from build123d import *

# Parameters (mm, degrees)
SKETCH2_W           = 203.2
SKETCH2_H           = 152.4
BOSS_EXTRUDE1_DEPTH = 152.4
SKETCH6_R           = 50.8
CUT_EXTRUDE2_DEPTH  = 228.6
SKETCH7_W           = 50.8
SKETCH7_H           = 50.8
CUT_EXTRUDE3_DEPTH  = 50.8
SKETCH5_W           = 50.8
SKETCH5_H           = 152.4
BOSS_EXTRUDE3_DEPTH = 50.8
SKETCH3_W           = 152.4
SKETCH3_H           = 101.6
CUT_EXTRUDE4_DEPTH  = 228.6


with BuildPart() as part:
    # Sketch2 → Boss-Extrude1 (new, symmetric)
    with BuildSketch(Plane(origin=(0, 0, 0), x_dir=(0, 0, -1), z_dir=(1, 0, 0))):
        Rectangle(SKETCH2_W, SKETCH2_H)
    extrude(amount=BOSS_EXTRUDE1_DEPTH, both=True)

    # Sketch6 → Cut-Extrude2 (cut)
    with BuildSketch(Plane.XY.offset(101.6)):
        with Locations((-25.4, 0)):
            Circle(SKETCH6_R)
    extrude(amount=-CUT_EXTRUDE2_DEPTH, mode=Mode.SUBTRACT)

    # Sketch7 → Cut-Extrude3 (cut)
    with BuildSketch(Plane.ZY.offset(152.4)):
        Rectangle(SKETCH7_W, SKETCH7_H)
    extrude(amount=-CUT_EXTRUDE3_DEPTH, mode=Mode.SUBTRACT)

    # Sketch5 → Boss-Extrude3 (add)
    with BuildSketch(Plane(origin=(0, 76.2, 0), x_dir=(1, 0, 0), z_dir=(0, 1, 0))):
        with Locations((101.6, 0)):
            Rectangle(SKETCH5_W, SKETCH5_H)
    extrude(amount=BOSS_EXTRUDE3_DEPTH)

    # Sketch3 → Cut-Extrude4 (cut)
    with BuildSketch(Plane(origin=(0, 76.2, 0), x_dir=(1, 0, 0), z_dir=(0, 1, 0))):
        with Locations((-25.4, 0)):
            Rectangle(SKETCH3_W, SKETCH3_H)
    extrude(amount=-CUT_EXTRUDE4_DEPTH, mode=Mode.SUBTRACT)


solid = part.part
CAD build for the part. Positions are in the model's coordinates, mm. A direction names the side the tool comes from. Coordinates: 2 decimals unless noted, no trailing zeros. Order: outer loops, then holes, each group sorted by start corner. A loop starts at its lowest first (then second) coordinate and runs counter-clockwise, first axis right, second up. Notation, with made-up numbers: (86, 48) -> (119, 48) arc R17 ccw to (119, 80) -> close; hole circle Ø11 at (-40, -35). An arc over 180 degrees is marked (long way). Answer in a Markdown table with one row per item.
1) Band-saw the part on D-D (y = 0). List the corners of the cut face in (x, z).
Check values:
| item | result |
|---|---|
| outline | (-152.4, -101.6) -> (-76.2, -101.6) -> (-76.2, -50.8) -> (-101.6, -50.8) -> (-101.6, -25.4) -> (-152.4, -25.4) -> close; (-152.4, 25.4) -> (-101.6, 25.4) -> (-101.6, 50.8) -> (-76.2, 50.8) -> (-76.2, 101.6) -> (-152.4, 101.6) -> close; (25.4, -101.6) -> (152.4, -101.6) -> (152.4, 101.6) -> (25.4, 101.6) -> (25.4, 50.8) -> (50.8, 50.8) -> (50.8, -50.8) -> (25.4, -50.8) -> close |
2) Band-saw the part on A-A (z = -3). List the corners of the cut face in (x, y).
Check values:
| item | result |
|---|---|
| outline | (-152.4, -76.2) -> (-101.6, -76.2) -> (-101.6, -25.4) -> (-152.4, -25.4) -> close; (-152.4, 25.4) -> (-101.6, 25.4) -> (-101.6, 76.2) -> (-152.4, 76.2) -> close; (50.8, -76.2) -> (152.4, -76.2) -> (152.4, 76.2) -> (127, 76.2) -> (127, 127) -> (76.2, 127) -> (76.2, 76.2) -> (50.8, 76.2) -> close |
3) Band-saw the part on C-C (z = 68). List the corners of the cut face in (x, y).
Check values:
| item | result |
|---|---|
| outline | (-152.4, -76.2) -> (152.4, -76.2) -> (152.4, 76.2) -> (127, 76.2) -> (127, 127) -> (76.2, 127) -> (76.2, 76.2) -> (-152.4, 76.2) -> close; hole circle Ø101.6 at (-25.4, 0) |
4) Band-saw the part on B-B (x = -96). List the corners of the cut face in (y, z), and give its area (3 significant figures).
Check values:
| item | result |
|---|---|
| outline | (-76.2, -101.6) -> (76.2, -101.6) -> (76.2, -50.8) -> (-76.2, -50.8) -> close; (-76.2, 50.8) -> (76.2, 50.8) -> (76.2, 101.6) -> (-76.2, 101.6) -> close |
| area | 15,500 mm2 |
5) Drill centre lines: line 1 (X direction, y = -34.5, z = 1.5); line 2 (Z direction, x = 41.5, y = -66); line 3 (Y direction, x = -25.4, z = -81.5). Where is each one in solid material? Low to high.
Check values:
| item | result |
|---|---|
| line 1 | -152.4 to -101.6, 50.8 to 152.4 |
| line 2 | -101.6 to -50.8, 50.8 to 101.6 |
| line 3 | -76.2 to -50.8, 50.8 to 76.2 |
6) Mould opens along X. For faces 1 (the face through (23.054, 15.259, 76.556)), 2 (the face through (152.4, 1, 1)), 3 (the face through (36, -1, 101.6)) say: pulls with the +X half, pulls with the -X half, needs draft (parallel to the pull), parting line crosses it, or undercut.
Check values:
| item | result |
|---|---|
| face 1 | undercut |
| face 2 | pulls with the +X half |
| face 3 | needs draft |
7) Flat gauge pins, fed straight in: P1, Ø10, axis at y = 101, z = 40.5, coming from the +X side; P2, Ø15, axis at y = 95, z = 27.5, coming from the -X side; P3, Ø15, axis at x = 106, y = 95, coming from the -Z side. Where does each tip first touch, or does it go through?
Check values:
| item | result |
|---|---|
| P1 | x = 127 |
| P2 | x = 76.2 |
| P3 | z = -76.2 |
8) Which spindle directions (+Z, -Z, +X, -X, +Y, -Y) get a long thin tool onto all of the face, cutting with end or side? Do faces 4 (the face through (101, 101, -76.2)), 5 (the face through (-127, 0, 25.4)), 6 (the face through (76.2, 101, 1)), 7 (the face through (-77, 1, -50.8)), 8 (the face through (127, 101, 1)). Say none if no direction does.
Check values:
| item | result |
|---|---|
| face 4 | -Z, +X, -X, +Y |
| face 5 | -X |
| face 6 | +Z, -Z, -X, +Y |
| face 7 | +Y, -Y |
| face 8 | +Z, -Z, +X, +Y |
